Autodesk Inventor part; units mm, degrees
ref_plane "center_XY" through (0, 0, 0) normal (1, 0, 0) x (0, 0, -1)
ref_plane "center_YZ" through (0, 0, 0) normal (0, 0, -1) x (0, 1, 0)
ref_plane "center_ZX" through (0, 0, 0) normal (0, 1, 0) x (1, 0, 0)
sketch "Sketch_4" plane through (0, 0, 0) normal (0, 0, 1) x (1, 0, 0)
  line L0 (4, 0) -> (0, 0)
  line L1 (0, 4.8586) -> (0, 4.35)
  line L2 (0, 4.35) -> (0.36, 4.35)
  line L3 (0.36, 4.35) -> (0.36, 4.125)
  line L4 (0.36, 4.125) -> (1.6031, 4.125)
  arc A0 (2.3969, 4.125) -> (1.6031, 4.125) centre (2, 3.675) ccw
  line L5 (2.3969, 4.125) -> (3.64, 4.125)
  line L6 (3.64, 4.125) -> (3.64, 4.35)
  line L7 (3.64, 4.35) -> (4, 4.35)
  line L8 (4, 4.35) -> (4, 4.8586)
  line L9 (4, 4.8586) -> (3.8586, 5)
  line L10 (3.8586, 5) -> (0.1414, 5)
  line L11 (0.1414, 5) -> (0, 4.8586)
revolve "Revolution1" add sketch "Sketch_4" angle 360 about axis through (4, 0, 0) along (1, 0, 0)
ref_plane "center_XY" through (0, 0, 0) normal (1, 0, 0) x (0, 0, -1)
ref_plane "center_YZ" through (0, 0, 0) normal (0, 0, -1) x (0, 1, 0)
ref_plane "center_ZX" through (0, 0, 0) normal (0, 1, 0) x (1, 0, 0)
ref_plane "or_1_1_XY" through (2, 3.675, 0) normal (1, 0, 0) x (0, 0, -1)
ref_plane "or_1_1_YZ" through (2, 3.675, 0) normal (0, 0, -1) x (0, 1, 0)
ref_plane "or_1_1_ZX" through (2, 3.675, 0) normal (0, 1, 0) x (1, 0, 0)
ref_plane "or_1_10_XY" through (2, 2.9731, -2.1601) normal (1, 0, 0) x (0, 0, -1)
ref_plane "or_1_10_YZ" through (2, 2.9731, -2.1601) normal (0, 0, -1) x (0, 1, 0)
ref_plane "or_1_10_ZX" through (2, 2.9731, -2.1601) normal (0, 1, 0) x (1, 0, 0)
ref_plane "or_1_2_XY" through (2, 2.9731, 2.1601) normal (1, 0, 0) x (0, 0, -1)
ref_plane "or_1_2_YZ" through (2, 2.9731, 2.1601) normal (0, 0, -1) x (0, 1, 0)
ref_plane "or_1_2_ZX" through (2, 2.9731, 2.1601) normal (0, 1, 0) x (1, 0, 0)
ref_plane "or_1_3_XY" through (2, 1.1356, 3.4951) normal (1, 0, 0) x (0, 0, -1)
ref_plane "or_1_3_YZ" through (2, 1.1356, 3.4951) normal (0, 0, -1) x (0, 1, 0)
ref_plane "or_1_3_ZX" through (2, 1.1356, 3.4951) normal (0, 1, 0) x (1, 0, 0)
ref_plane "or_1_4_XY" through (2, -1.1356, 3.4951) normal (1, 0, 0) x (0, 0, -1)
ref_plane "or_1_4_YZ" through (2, -1.1356, 3.4951) normal (0, 0, -1) x (0, 1, 0)
ref_plane "or_1_4_ZX" through (2, -1.1356, 3.4951) normal (0, 1, 0) x (1, 0, 0)
ref_plane "or_1_5_XY" through (2, -2.9731, 2.1601) normal (1, 0, 0) x (0, 0, -1)
ref_plane "or_1_5_YZ" through (2, -2.9731, 2.1601) normal (0, 0, -1) x (0, 1, 0)
ref_plane "or_1_5_ZX" through (2, -2.9731, 2.1601) normal (0, 1, 0) x (1, 0, 0)
ref_plane "or_1_6_XY" through (2, -3.675, 0) normal (1, 0, 0) x (0, 0, -1)
ref_plane "or_1_6_YZ" through (2, -3.675, 0) normal (0, 0, -1) x (0, 1, 0)
ref_plane "or_1_6_ZX" through (2, -3.675, 0) normal (0, 1, 0) x (1, 0, 0)
ref_plane "or_1_7_XY" through (2, -2.9731, -2.1601) normal (1, 0, 0) x (0, 0, -1)
ref_plane "or_1_7_YZ" through (2, -2.9731, -2.1601) normal (0, 0, -1) x (0, 1, 0)
ref_plane "or_1_7_ZX" through (2, -2.9731, -2.1601) normal (0, 1, 0) x (1, 0, 0)
ref_plane "or_1_8_XY" through (2, -1.1356, -3.4951) normal (1, 0, 0) x (0, 0, -1)
ref_plane "or_1_8_YZ" through (2, -1.1356, -3.4951) normal (0, 0, -1) x (0, 1, 0)
ref_plane "or_1_8_ZX" through (2, -1.1356, -3.4951) normal (0, 1, 0) x (1, 0, 0)
ref_plane "or_1_9_XY" through (2, 1.1356, -3.4951) normal (1, 0, 0) x (0, 0, -1)
ref_plane "or_1_9_YZ" through (2, 1.1356, -3.4951) normal (0, 0, -1) x (0, 1, 0)
ref_plane "or_1_9_ZX" through (2, 1.1356, -3.4951) normal (0, 1, 0) x (1, 0, 0)
ref_plane "outer_XY" through (4, 0, 0) normal (1, 0, 0) x (0, 0, -1)
ref_plane "outer_YZ" through (4, 0, 0) normal (0, 0, -1) x (0, 1, 0)
ref_plane "outer_ZX" through (4, 0, 0) normal (0, 1, 0) x (1, 0, 0)
properties part number "WML5010ZZ Outer ring"
Work out the finished part from the listing and answer in its coordinate system (mm). A direction names the side the tool comes from. Give positions to 0.01 mm unless a question says otherwise; leave off trailing zeros. Write each loop counter-clockwise with the first axis right and the second up, starting at its lowest first coordinate (ties: lowest second). Pieces come first, ordered by that corner, then holes. Notation, with made-up numbers: (14, 53.25) -> (71, 53.25) arc R6 ccw to (71, 61.25) -> close; hole circle Ø9 at (13, 57). An arc over 180 degrees is marked (long way). Write item = value, one per line.
Q1. Flat-ended cylindrical pins translate along their axes: pin 1 Ø4.5 at (y, z) = (0, -1.5) entering from +X; pin 2 Ø2 at (x, z) = (2, 1.5) entering from -Y; pin 3 Ø2 at (x, y) = (2.5, -2) entering from -Z; pin 4 Ø2 at (x, z) = (2, -4) entering from +Y. Find the tip coordinate at first contact, or state that the pin passes through.
Computed values:
pin_1 = through
pin_2 = -4.97
pin_3 = -4.9
pin_4 = 4
Q2. Section D-D on x = 2.2 is taken. Determine the outline of the cut face in (y, z).
Computed values:
outline = circle Ø10 at (0, 0); hole circle Ø8.48 at (0, 0)
Q3. Consider line 1 along Z through (x, y) = (1.25, 0) (3 decimals); line 2 along Z through (x, y) = (3.95, 0); line 3 along Y through (x, z) = (1.75, -2.75). Determine where each line is inside the solid, lowest interval first.
Computed values:
line_1 = -5 to -4.125, 4.125 to 5
line_2 = -4.91 to -4.35, 4.35 to 4.91
line_3 = -4.18 to -3.2, 3.2 to 4.18
Q4. Section A-A on y = 0 is taken. Determine the outline of the cut face in (x, z) (3 decimals), and give its area (3 significant figures).
Computed values:
outline = (0, -4.859) -> (0.141, -5) -> (3.859, -5) -> (4, -4.859) -> (4, -4.35) -> (3.64, -4.35) -> (3.64, -4.125) -> (2.397, -4.125) arc R0.6 cw to (1.603, -4.125) -> (0.36, -4.125) -> (0.36, -4.35) -> (0, -4.35) -> close; (0, 4.35) -> (0.36, 4.35) -> (0.36, 4.125) -> (1.603, 4.125) arc R0.6 cw to (2.397, 4.125) -> (3.64, 4.125) -> (3.64, 4.35) -> (4, 4.35) -> (4, 4.859) -> (3.859, 5) -> (0.141, 5) -> (0, 4.859) -> close
area = 6.47 mm^2
Q5. For a pull along Y with two mould halves and no side action, classify faces 1 (the cylindrical face through (3.823, -0.943, -4.247)), 2 (the cylindrical face through (1.97, -1.08, 4.88)) as pulls with the +Y half, pulls with the -Y half, needs draft (parallel to the pull), parting line crosses it, or undercut.
Computed values:
face_1 = undercut
face_2 = parting line crosses it
Q6. Section C-C on x = 3.45 is taken. Determine the outline of the cut face in (y, z) (3 decimals), and give its area (3 significant figures).
Computed values:
outline = circle Ø10 at (0, 0); hole circle Ø8.25 at (0, 0)
area = 25.1 mm^2
Q7. A tool of negligible diameter and unlimited length cuts with its end or side. For faces 3 (the cylindrical face through (0.183, -0.943, -4.247)), 4 (the cylindrical face through (1, 3.8, -1.6)), from which of +Z, -Z, +X, -X, +Y, -Y can it reach the whole face along a straight path? Write none if from no direction.
Computed values:
face_3 = -X
face_4 = +X, -X
